Here's the drawing with two shaded views (mm, measured from the low corner). I have some questions. A direction names the side the tool comes from. Coordinates: 2 decimals unless noted, no trailing zeros. Write each loop counter-clockwise with the first axis right and the second up, starting at its lowest first coordinate (ties: lowest second). Pieces come first, ordered by that corner, then holes.
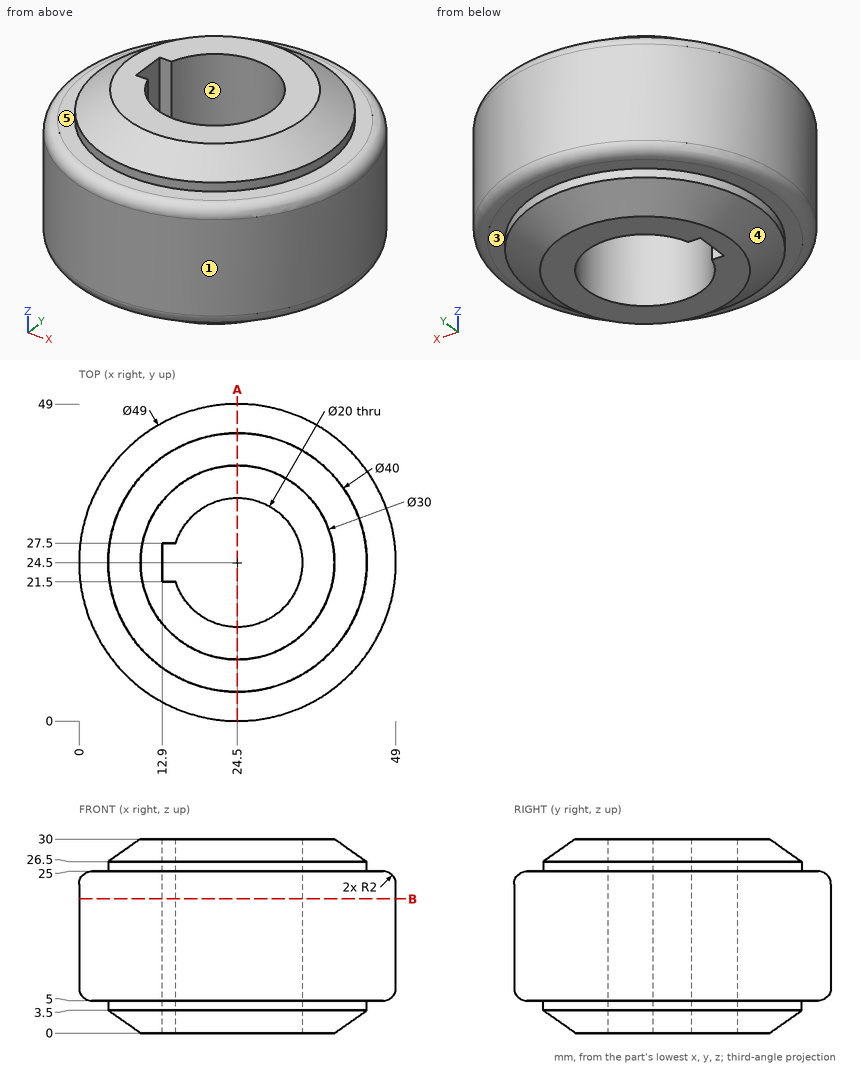
1. On a 3-axis mill with a long thin cutter (end or side, diameter ignored), from which of +Z, -Z, +X, -X, +Y, -Y can I reach the whole of each face in a straight line? I mean the marked faces 4 and 5. Say none if no direction works.
Verdict:
face 4: -Z
face 5: +Z
2. Please list where these lines run through material, in increasing order: line 1 along Y through (x, z) = (24.5, 15); line 2 along Y through (x, z) = (30, 17.5); line 3 along Z through (x, y) = (38, 40).
Verdict:
line 1: y = 0 to 14.5, 34.5 to 49
line 2: y = 0.63 to 16.15, 32.85 to 48.37
line 3: z = 5 to 25
3. I want a section at B-B on z = 20.75. Please give me the cut outline in (x, y).
Verdict:
outline: circle Ø49 at (24.5, 24.5); hole (12.9, 21.5) - (14.96, 21.5) arc R10 ccw (long way) to (14.96, 27.5) - (12.9, 27.5) - close
4. If we mould it in two halves opening along Y, with no side actions, what happens to the marked faces 1, 2 and 3? For each: pulls with the +Y half, pulls with the -Y half, needs draft (parallel to the pull), parting line crosses it, or undercut.
Verdict:
face 1: parting line crosses it
face 2: undercut
face 3: needs draft
5. I want a section at A-A on x = 24.5. Please give me the cut outline in (y, z), plus the area to 3 significant figures.
Verdict:
outline: (0, 7) arc R2 ccw to (2, 5) - (4.5, 5) - (4.5, 3.5) - (9.5, 0) - (14.5, 0) - (14.5, 30) - (9.5, 30) - (4.5, 26.5) - (4.5, 25) - (2, 25) arc R2 ccw to (0, 23) - close; (34.5, 0) - (39.5, 0) - (44.5, 3.5) - (44.5, 5) - (47, 5) arc R2 ccw to (49, 7) - (49, 23) arc R2 ccw to (47, 25) - (44.5, 25) - (44.5, 26.5) - (39.5, 30) - (34.5, 30) - close
area: 742 mm2
6. For pin 1 (6 mm diameter, centred on x = 10.5, y = 12.5, fed in from +Z); pin 2 (12 mm diameter, centred on x = 23.5, z = 12.5, fed in from -Y); pin 3 (0.6 mm diameter, centred on x = 14, z = 17.5, fed in from +Y); pin 4 (16 mm diameter, centred on x = 24.5, y = 24.5, fed in from -Z), each with a flat end and sliding along its axis, tell me the tip position at first contact or that it passes through.
Verdict:
pin 1: stops at z = 29.69
pin 2: stops at y = 0
pin 3: stops at y = 46.78
pin 4: passes through
